The model under review builds one solid part; all positions refer to its coordinate system, in mm. A direction names the side the tool comes from. Round coordinates to 2 decimals unless told otherwise and drop trailing zeros. Write each loop counter-clockwise with the first axis right and the second up, starting at its lowest first coordinate (ties: lowest second). Pieces come first, ordered by that corner, then holes. Notation, with made-up numbers: M 55.5,-19.5 L 110.5,-19.5 A28 ccw 110.5,17.5 Z; hole C 59.5,0 d9. An arc over 180 degrees is marked long. Write item = value, one per line. Start each with the question number.
Item 1: Take a section at D-D, the plane x = -1357. Give the boundary of the cut face in (y, z).
Item 2: Take a section at C-C, the plane z = 2.2. Give the boundary of the cut face in (x, y).
Item 3: Take a section at B-B, the plane x = -1342. Give the boundary of the cut face in (y, z), plus the area to 3 significant figures.
Item 4: Tool access review of faces 5 (the flat face through (-1332, 88.9, 1)), 6 (the cylindrical face through (-1319.397, 91.583, 1.479)), 7 (the flat face through (-1344, 96.861, 1)), 8 (the flat face through (-1351.28, 97, 1)): name each direction out of +Z, -Z, +X, -X, +Y, -Y from which nothing blocks a thin tool from reaching the whole face with its end or side.
Item 5: The part is to be moulded in two halves that separate along Y. For faces 1 (the flat face through (-1341.167, 99, 1)), 2 (the flat face through (-1346.167, 95, 1)), 3 (the flat face through (-1346, 100.515, 1)), 4 (the flat face through (-1338, 93.9, 1)), say which applies: +Y half, -Y half, draft (parallel to the pull), parting line (faces both ways), or undercut.
Item 6: To check wall thickness, follow line 1 along Y through (x, z) = (-1359, 1.45); line 2 along X through (y, z) = (94.5, 0.95); line 3 along X through (y, z) = (85, 1.6). State the ranges of each line that lie inside material, in increasing order.
Item 7: For pin 1 Ø0.9 at (x, z) = (-1332, 2) entering from -Y; pin 2 Ø1.5 at (y, z) = (96.5, 2) entering from -X; pin 3 Ø0.9 at (x, z) = (-1356, 2) entering from +Y; pin 4 Ø5 at (x, y) = (-1358, 80.5) entering from +Z, all flat-tipped, find the tip position at first contact; note any pin that passes through.
Item 8: Take a section at A-A, the plane y = 95.75. Give the boundary of the cut face in (x, z).
from build123d import *

# Parameters (mm, degrees)
BASE_EXTRUDE_DEPTH = 3


with BuildPart() as part:
    # Sketch1 → Base-Extrude (new body)
    with BuildSketch(Plane.XY):
        with BuildLine():
            Line((-1351.280186532, 100.515097097), (-1341.166910128, 100.515097097))
            Line((-1341.166910128, 100.515097097), (-1341.166910128, 96.861073329))
            Line((-1341.166910128, 96.861073329), (-1346.166910128, 96.861073329))
            Line((-1346.166910128, 96.861073329), (-1346.166910128, 93.899820126))
            Line((-1346.166910128, 93.899820126), (-1328.72354833, 93.899820126))
            ThreePointArc((-1328.72354833, 93.899820126), (-1319.393421311, 91.399820126), (-1328.72354833, 88.899820126))
            Line((-1328.72354833, 88.899820126), (-1336.22354833, 88.899820126))
            Line((-1336.22354833, 88.899820126), (-1336.22354833, 82.793437515))
            ThreePointArc((-1336.22354833, 82.793437515), (-1346.22354833, 76.504450604), (-1356.22354833, 82.793437515))
            Line((-1356.22354833, 82.793437515), (-1356.22354833, 88.899820126))
            Line((-1356.22354833, 88.899820126), (-1363.72354833, 88.899820126))
            ThreePointArc((-1363.72354833, 88.899820126), (-1373.053675349, 91.399820126), (-1363.72354833, 93.899820126))
            Line((-1363.72354833, 93.899820126), (-1351.280186532, 93.899820126))
            Line((-1351.280186532, 93.899820126), (-1351.280186532, 100.515097097))
        make_face()
    extrude(amount=BASE_EXTRUDE_DEPTH)


solid = part.part
Response values:
q1.outline = M 88.9,0 L 93.9,0 L 93.9,3 L 88.9,3 Z
q2.outline = M -1363.72,88.9 L -1356.22,88.9 L -1356.22,82.79 A11.09 ccw -1336.22,82.79 L -1336.22,88.9 L -1328.72,88.9 A5 ccw long -1328.72,93.9 L -1346.17,93.9 L -1346.17,96.86 L -1341.17,96.86 L -1341.17,100.52 L -1351.28,100.52 L -1351.28,93.9 L -1363.72,93.9 A5 ccw long Z
q3.outline = M 77.34,0 L 93.9,0 L 93.9,3 L 77.34,3 Z; M 96.86,0 L 100.52,0 L 100.52,3 L 96.86,3 Z
q3.area = 60.6 mm2
q4.face_5 = +Z, -Z, -Y
q4.face_6 = +Z, -Z
q4.face_7 = +Z, -Z, +X
q4.face_8 = +Z, -Z, +Y
q5.face_1 = draft
q5.face_2 = undercut
q5.face_3 = +Y half
q5.face_4 = undercut
q6.line_1 = 88.9 to 93.9
q6.line_2 = -1371.98 to -1364.13, -1351.28 to -1346.17, -1328.32 to -1320.47
q6.line_3 = -1356.22 to -1336.22
q7.pin_1 = 88.9
q7.pin_2 = -1370.52
q7.pin_3 = 93.9
q7.pin_4 = through
q8.outline = M -1370.52,0 L -1365.59,0 L -1365.59,3 L -1370.52,3 Z; M -1351.28,0 L -1346.17,0 L -1346.17,3 L -1351.28,3 Z; M -1326.86,0 L -1321.93,0 L -1321.93,3 L -1326.86,3 Z
